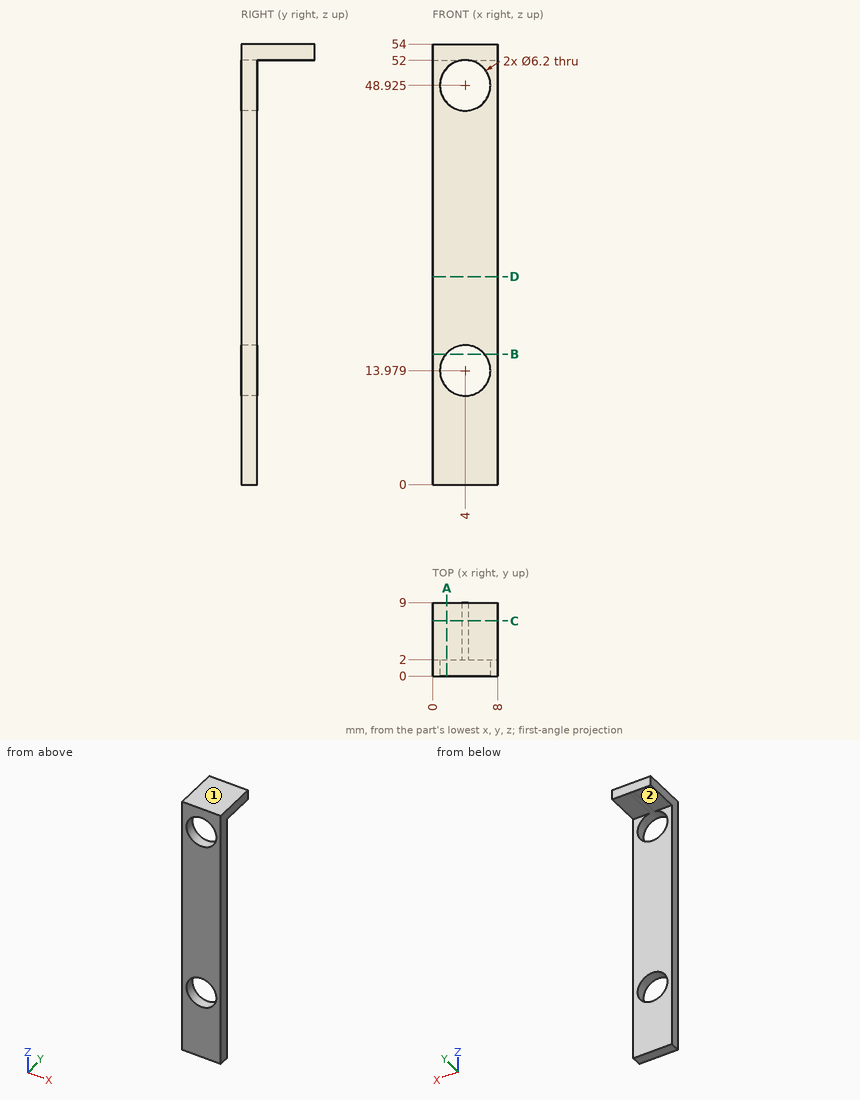
The figure shows three views and two pictorial views of one solid part (mm, origin at its lowest corner). Answer the questions. A direction names the side the tool comes from. Round coordinates to 2 decimals unless told otherwise and drop trailing zeros. Order: outer loops, then holes, each group sorted by start corner. A loop starts at its lowest first (then second) coordinate and runs counter-clockwise, first axis right, second up.
Q1. A cutting plane is placed at D-D, the plane z = 25.5. Determine the outline of the cut face in (x, y), then the cut area to 3 significant figures.
Solution:
outline: (0, 0) - (8, 0) - (8, 2) - (0, 2) - close
area: 16.0 mm2
Q2. A cutting plane is placed at C-C, the plane y = 6.75. Determine the outline of the cut face in (x, z) (1 decimal).
Solution:
outline: (0, 52) - (3.6, 52) arc R3.1 cw to (4.4, 52) - (8, 52) - (8, 54) - (0, 54) - close
Q3. A cutting plane is placed at A-A, the plane x = 1.75. Determine the outline of the cut face in (y, z).
Solution:
outline: (0, 0) - (2, 0) - (2, 11.85) - (0, 11.85) - close; (0, 16.11) - (2, 16.11) - (2, 46.79) - (0, 46.79) - close; (0, 51.06) - (2, 51.06) - (2, 52) - (9, 52) - (9, 54) - (0, 54) - close
Q4. Find the intervals of material crossed by line 1 along Z through (x, y) = (4, 0.7) (1 decimal); line 2 along Z through (x, y) = (6.25, 5.75); line 3 along Y through (x, z) = (1.5, 24.5), in increasing order.
Solution:
line 1: z = 0 to 10.9, 17.1 to 45.8, 52 to 54
line 2: z = 52 to 54
line 3: y = 0 to 2
Q5. A cutting plane is placed at B-B, the plane z = 16. Determine the outline of the cut face in (x, y).
Solution:
outline: (0, 0) - (1.65, 0) - (1.65, 2) - (0, 2) - close; (6.35, 0) - (8, 0) - (8, 2) - (6.35, 2) - close
Q6. Given pin 1 Ø3 at (x, z) = (3.5, 47) entering from +Y; pin 2 Ø3.5 at (x, z) = (4, 13.98) entering from -Y; pin 3 Ø1 at (x, y) = (1.5, 5) entering from -Z, each flat-ended and moving along its own axis, determine where each tip first touches the part or whether it passes through.
Solution:
pin 1: stops at y = 2
pin 2: passes through
pin 3: stops at z = 52
Q7. A tool of negligible diameter and unlimited length cuts with its end or side. For the marked faces 1 and 2, from which of +Z, -Z, +X, -X, +Y, -Y can it reach the whole face along a straight path? Write none if from no direction.
Solution:
face 1: +Z, +X, -X, +Y, -Y
face 2: -Z, +X, -X, +Y
